```python
from build123d import *

# Parameters (mm, degrees)
F0_W     = 508
F0_H     = 50.8
F1_DEPTH = 19.05
F3_DEPTH = 12.7
F5_DEPTH = 25.4


with BuildPart() as f1:
    # F0 (on Front) → F1 (new body)
    with BuildSketch(Plane.XZ):
        with Locations((254, 25.4)):
            Rectangle(F0_W, F0_H)
    extrude(amount=F1_DEPTH)

    # F2 (on face) → F3 (cut)
    with BuildSketch(Plane.XZ.offset(19.05)):
        with BuildLine():
            Line((480.695, 32.004), (27.305, 32.004))
            ThreePointArc((27.305, 32.004), (25.059936, 31.074064), (24.13, 28.829))
            Line((24.13, 28.829), (24.13, 21.971))
            ThreePointArc((24.13, 21.971), (25.059936, 19.725936), (27.305, 18.796))
            Line((27.305, 18.796), (480.695, 18.796))
            ThreePointArc((480.695, 18.796), (482.940064, 19.725936), (483.87, 21.971))
            Line((483.87, 21.971), (483.87, 28.829))
            ThreePointArc((483.87, 28.829), (482.940064, 31.074064), (480.695, 32.004))
        make_face()
    extrude(amount=-F3_DEPTH, mode=Mode.SUBTRACT)

    # F4 (on face) → F5 (cut)
    with BuildSketch(Plane.XZ.offset(19.05)):
        with BuildLine():
            Line((473.075, 32.004), (34.925, 32.004))
            ThreePointArc((34.925, 32.004), (32.679936, 31.074064), (31.75, 28.829))
            Line((31.75, 28.829), (31.75, 21.971))
            ThreePointArc((31.75, 21.971), (32.679936, 19.725936), (34.925, 18.796))
            Line((34.925, 18.796), (473.075, 18.796))
            ThreePointArc((473.075, 18.796), (475.320064, 19.725936), (476.25, 21.971))
            Line((476.25, 21.971), (476.25, 28.829))
            ThreePointArc((476.25, 28.829), (475.320064, 31.074064), (473.075, 32.004))
        make_face()
    extrude(amount=-F5_DEPTH, mode=Mode.SUBTRACT)


solid = f1.part
```
The listing builds one solid part. Answer for the finished solid, in the listing's coordinates (mm). A direction names the side the tool comes from. Round coordinates to 2 decimals unless told otherwise and drop trailing zeros. Loops run counter-clockwise (first coordinate to the right, second up) from the corner with the lowest first, then second, coordinate; pieces in that order, holes last.
1) A cutting plane is placed at A-A on y = -3.25. Determine the outline of the cut face in (x, z) (3 decimals).
Outcome:
outline: (0, 0) - (508, 0) - (508, 50.8) - (0, 50.8) - close; hole (31.75, 21.971) arc R3.175 ccw to (34.925, 18.796) - (473.075, 18.796) arc R3.175 ccw to (476.25, 21.971) - (476.25, 28.829) arc R3.175 ccw to (473.075, 32.004) - (34.925, 32.004) arc R3.175 ccw to (31.75, 28.829) - close
2) Given P1, Ø3, axis at x = 477.5, z = 22.5, coming from the -Y side, flat-ended and moving along its own axis, determine where the tip first touches the part or whether it passes through.
Outcome:
P1: stops at y = -6.35
3) For a pull along Z with two mould halves and no side action, classify faces 3 (the face through (0, -9, 25)), 4 (the face through (250, -9, 50.8)), 5 (the face through (28, -6.35, 25)) as released by +Z, released by -Z, zero draft, split by the parting line, or undercut.
Outcome:
face 3: zero draft
face 4: released by +Z
face 5: undercut
4) For faces 1 (the face through (250, -19.05, 14)), 2 (the face through (480, -6.35, 25)), determine the directions among +Z, -Z, +X, -X, +Y, -Y from which every point of the face is accessible in a straight line to the end or side of a thin tool.
Outcome:
face 1: +Z, -Z, +X, -X, -Y
face 2: -Y
5) A cutting plane is placed at B-B on x = 65. Determine the outline of the cut face in (y, z), plus the area to 3 significant figures.
Outcome:
outline: (-19.05, 0) - (0, 0) - (0, 18.8) - (-19.05, 18.8) - close; (-19.05, 32) - (0, 32) - (0, 50.8) - (-19.05, 50.8) - close
area: 716 mm2
6) Consider line 1 (Z direction, x = 47.5, y = -14.5); line 2 (X direction, y = -16.5, z = 22.5); line 3 (X direction, y = -3, z = 27). Determine where each line is inside the solid, lowest interval first.
Outcome:
line 1: z = 0 to 18.8, 32 to 50.8
line 2: x = 0 to 24.13, 483.87 to 508
line 3: x = 0 to 31.75, 476.25 to 508
